For this review, take the finished solid that the model builds, in its own axes (mm). A direction names the side the tool comes from. Give positions to 0.01 mm unless a question says otherwise; leave off trailing zeros. Write each loop counter-clockwise with the first axis right and the second up, starting at its lowest first coordinate (ties: lowest second). Pieces come first, ordered by that corner, then holes. Notation, with made-up numbers: (72, 18) -> (87, 18) arc R26 ccw to (87, 52) -> close; hole circle Ø1 at (-26.5, 67.5). An arc over 180 degrees is marked (long way). Write item = value, one per line.
```python
from build123d import *

# Parameters (mm, degrees)
SZKIC1_W                    = 175
SZKIC1_H                    = 118.3
DODANIE_WYCI_GNI_CIE1_DEPTH = 5
SZKIC2_W                    = 5
SZKIC2_H                    = 118.3
DODANIE_WYCI_GNI_CIE2_DEPTH = 25
SZKIC3_W                    = 5
SZKIC3_H                    = 118.3
DODANIE_WYCI_GNI_CIE3_DEPTH = 100
SZKIC4_W                    = 165
SZKIC4_H                    = 5
DODANIE_WYCI_GNI_CIE4_DEPTH = 25
SZKIC5_W                    = 165
SZKIC5_H                    = 5
DODANIE_WYCI_GNI_CIE5_DEPTH = 25
WYTNIJ_WYCI_GNI_CIE1_REACH  = 214.482
SZKIC7_W                    = 14
SZKIC7_H                    = 17.1
WYTNIJ_WYCI_GNI_CIE2_REACH  = 214.482
SZKIC8_W                    = 10.9
SZKIC8_H                    = 17.1


with BuildPart() as part:
    # Szkic1 → Dodanie-wyciągnięcie1 (new body)
    with BuildSketch(Plane(origin=(0, 0, 0), x_dir=(1, 0, 0), z_dir=(0, 1, 0))):
        Rectangle(SZKIC1_W, SZKIC1_H)
    extrude(amount=DODANIE_WYCI_GNI_CIE1_DEPTH)

    # Szkic2 → Dodanie-wyciągnięcie2 (add)
    with BuildSketch(Plane(origin=(0, 5, 0), x_dir=(1, 0, 0), z_dir=(0, 1, 0))):
        with Locations((-85, 0)):
            Rectangle(SZKIC2_W, SZKIC2_H)
    extrude(amount=DODANIE_WYCI_GNI_CIE2_DEPTH)

    # Szkic3 → Dodanie-wyciągnięcie3 (add)
    with BuildSketch(Plane(origin=(0, 5, 0), x_dir=(1, 0, 0), z_dir=(0, 1, 0))):
        with Locations((85, 0)):
            Rectangle(SZKIC3_W, SZKIC3_H)
    extrude(amount=DODANIE_WYCI_GNI_CIE3_DEPTH)

    # Szkic4 → Dodanie-wyciągnięcie4 (add)
    with BuildSketch(Plane(origin=(0, 5, 0), x_dir=(1, 0, 0), z_dir=(0, 1, 0))):
        with Locations((0, -56.65)):
            Rectangle(SZKIC4_W, SZKIC4_H)
    extrude(amount=DODANIE_WYCI_GNI_CIE4_DEPTH)

    # Szkic5 → Dodanie-wyciągnięcie5 (add)
    with BuildSketch(Plane(origin=(0, 5, 0), x_dir=(1, 0, 0), z_dir=(0, 1, 0))):
        with Locations((0, 56.65)):
            Rectangle(SZKIC5_W, SZKIC5_H)
    extrude(amount=DODANIE_WYCI_GNI_CIE5_DEPTH)

    # Szkic7 → Wytnij-wyciągnięcie1 (cut, up to next)
    with BuildSketch(Plane(origin=(87.5, 0, 0), x_dir=(0, 0, -1), z_dir=(1, 0, 0)), mode=Mode.PRIVATE) as wytnij_wyci_gni_cie1_sk1:
        with Locations((16.45, 13.55)):
            Rectangle(SZKIC7_W, SZKIC7_H)
    wytnij_wyci_gni_cie1_tool1 = extrude(wytnij_wyci_gni_cie1_sk1.sketch, amount=-WYTNIJ_WYCI_GNI_CIE1_REACH, mode=Mode.PRIVATE) & part.part
    add(wytnij_wyci_gni_cie1_tool1.solids().sort_by_distance((87.5, 13.55, -16.45))[0], mode=Mode.SUBTRACT)

    # Szkic8 → Wytnij-wyciągnięcie2 (cut, up to next)
    with BuildSketch(Plane(origin=(87.5, 0, 0), x_dir=(0, 0, -1), z_dir=(1, 0, 0)), mode=Mode.PRIVATE) as wytnij_wyci_gni_cie2_sk1:
        with Locations((46.4, 13.55)):
            Rectangle(SZKIC8_W, SZKIC8_H)
    wytnij_wyci_gni_cie2_tool1 = extrude(wytnij_wyci_gni_cie2_sk1.sketch, amount=-WYTNIJ_WYCI_GNI_CIE2_REACH, mode=Mode.PRIVATE) & part.part
    add(wytnij_wyci_gni_cie2_tool1.solids().sort_by_distance((87.5, 13.55, -46.4))[0], mode=Mode.SUBTRACT)


solid = part.part
```
(1) To check wall thickness, follow probe 1 along Z at (x, y) = (77.5, 8); probe 2 along X at (y, z) = (6.5, 16); probe 3 along Y at (x, z) = (-64, 45.5). State the ranges of each line that lie inside material, in increasing order.
Answers below:
probe_1 = -59.15 to -54.15, 54.15 to 59.15
probe_2 = -87.5 to -82.5, 82.5 to 87.5
probe_3 = 0 to 5
(2) Take a section at D-D (y = 93.5). Write out the cut boundary in (x, z).
Answers below:
outline = (82.5, -59.15) -> (87.5, -59.15) -> (87.5, 59.15) -> (82.5, 59.15) -> close
(3) The part is to be moulded in two halves that separate along Y. For faces 6 (the face through (87.5, 52, 1)), 7 (the face through (85, 22.1, -16)), 8 (the face through (-1, 0, -1)), say which applies: released by +Y, released by -Y, zero draft, split by the parting line, or undercut.
Answers below:
face_6 = zero draft
face_7 = undercut
face_8 = released by -Y
(4) For pin 1 (1.5 mm diameter, centred on x = 57.5, z = 30.5, fed in from +Y), flat-tipped, find the tip position at first contact; note if it passes through.
Answers below:
pin_1 = 5
(5) Tool access review of faces 1 (the face through (85, 105, -1)), 2 (the face through (-85, 30, 0)), 3 (the face through (-82.5, 17, 1)), 4 (the face through (85, 22.1, -46)), 5 (the face through (-87.5, 15, 1)): name each direction out of +Z, -Z, +X, -X, +Y, -Y from which nothing blocks a thin tool from reaching the whole face with its end or side.
Answers below:
face_1 = +Z, -Z, +X, -X, +Y
face_2 = +Z, -Z, -X, +Y
face_3 = +Y
face_4 = +X
face_5 = +Z, -Z, -X, +Y, -Y
(6) Take a section at C-C (x = -55). Write out the cut boundary in (y, z), plus the area to 4 significant figures.
Answers below:
outline = (0, -59.15) -> (30, -59.15) -> (30, -54.15) -> (5, -54.15) -> (5, 54.15) -> (30, 54.15) -> (30, 59.15) -> (0, 59.15) -> close
area = 841.5 mm^2
(7) Take a section at A-A (y = 16). Write out the cut boundary in (x, z), plus the area to 3 significant figures.
Answers below:
outline = (-87.5, -59.15) -> (87.5, -59.15) -> (87.5, -51.85) -> (82.5, -51.85) -> (82.5, -54.15) -> (-82.5, -54.15) -> (-82.5, 54.15) -> (82.5, 54.15) -> (82.5, -9.45) -> (87.5, -9.45) -> (87.5, 59.15) -> (-87.5, 59.15) -> close; (82.5, -40.95) -> (87.5, -40.95) -> (87.5, -23.45) -> (82.5, -23.45) -> close
area = 2,710 mm^2
(8) Take a section at B-B (z = 26). Write out the cut boundary in (x, y), plus the area to 3 significant figures.
Answers below:
outline = (-87.5, 0) -> (87.5, 0) -> (87.5, 105) -> (82.5, 105) -> (82.5, 5) -> (-82.5, 5) -> (-82.5, 30) -> (-87.5, 30) -> close
area = 1,500 mm^2
